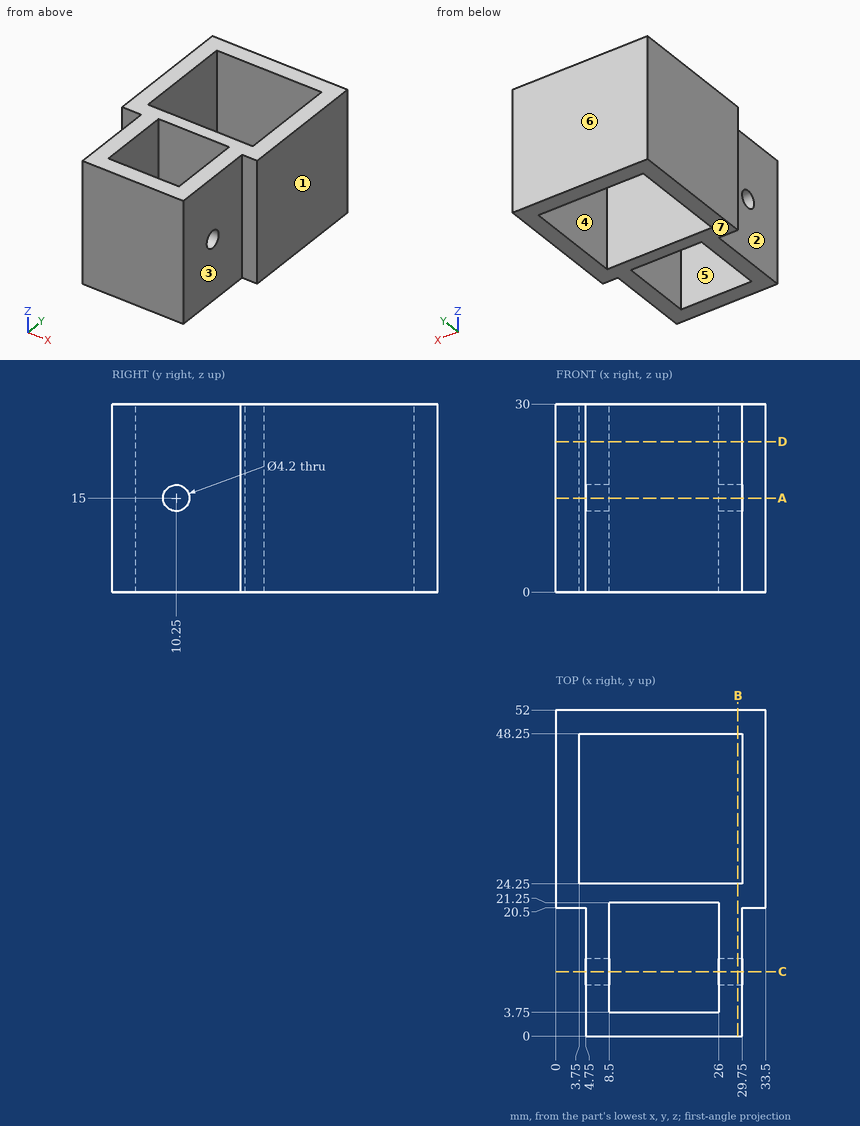
The figure shows three views and two pictorial views of one solid part (mm, origin at its lowest corner). Answer the questions. A direction names the side the tool comes from. Give positions to 0.01 mm unless a question says otherwise; leave off trailing zeros. Order: outer loops, then holes, each group sorted by start corner. A loop starts at its lowest first (then second) coordinate and runs counter-clockwise, first axis right, second up. Notation, with made-up numbers: M -6,-23 L 0,-23 A24 ccw 0,14 Z; hole C -38,5 d10. An arc over 180 degrees is marked long. Return JSON: item names as keys, results as strings.
1) Straight lines are drawn through the part: line 1 along Y through (x, z) = (10.5, 2.25); line 2 along X through (y, z) = (44.5, 27.5); line 3 along Z through (x, y) = (28.6, 10.25). For each, find the intervals that lie inside material, in ascending order. Write a range as [from, to].
Resolved:
{"line 1": "[0, 3.75], [21.25, 24.25], [48.25, 52]", "line 2": "[0, 3.75], [29.75, 33.5]", "line 3": "[0, 12.9], [17.1, 30]"}
2) Section D-D, the plane z = 24 is taken. Write down the section's boundary in (x, y), plus the area to 4 significant figures.
Resolved:
{"outline": "M 0,20.5 L 4.75,20.5 L 4.75,0 L 29.75,0 L 29.75,20.5 L 33.5,20.5 L 33.5,52 L 0,52 Z; hole M 3.75,24.25 L 29.75,24.25 L 29.75,48.25 L 3.75,48.25 Z; hole M 8.5,3.75 L 26,3.75 L 26,21.25 L 8.5,21.25 Z", "area": "637.5 mm^2"}
3) For a pull along Y with two mould halves and no side action, classify the marked faces 5, 6 and 7 as +Y half, -Y half, draft (parallel to the pull), parting line (faces both ways), or undercut.
Resolved:
{"face 5": "undercut", "face 6": "+Y half", "face 7": "draft"}
4) Section A-A, the plane z = 15 is taken. Write down the section's boundary in (x, y), plus the area to 3 significant figures.
Resolved:
{"outline": "M 0,20.5 L 4.75,20.5 L 4.75,12.35 L 8.5,12.35 L 8.5,21.25 L 26,21.25 L 26,12.35 L 29.75,12.35 L 29.75,20.5 L 33.5,20.5 L 33.5,52 L 0,52 Z; M 4.75,0 L 29.75,0 L 29.75,8.15 L 26,8.15 L 26,3.75 L 8.5,3.75 L 8.5,8.15 L 4.75,8.15 Z; hole M 3.75,24.25 L 29.75,24.25 L 29.75,48.25 L 3.75,48.25 Z", "area": "606 mm^2"}
5) A tool of negligible diameter and unlimited length cuts with its end or side. For the marked faces 1, 2, 3 and 4, from which of +Z, -Z, +X, -X, +Y, -Y can it reach the whole face along a straight path? Write none if from no direction.
Resolved:
{"face 1": "+Z, -Z, +X, +Y, -Y", "face 2": "+Z, -Z, -X, -Y", "face 3": "+Z, -Z, +X, -Y", "face 4": "+Z, -Z"}
6) Each of these flat-tipped pins is pushed along its axis until it touches: pin 1 (4 mm diameter, centred on y = 45, z = 13, fed in from -X); pin 2 (6.5 mm diameter, centred on y = 10.25, z = 15, fed in from +X); pin 3 (5 mm diameter, centred on y = 14.5, z = 13.5, fed in from -X); pin 4 (1.1 mm diameter, centred on x = 32, z = 12.5, fed in from -Y). Where does it stop, or does it pass through?
Resolved:
{"pin 1": "x = 0", "pin 2": "x = 29.75", "pin 3": "x = 4.75", "pin 4": "y = 20.5"}
7) Section B-B, the plane x = 29 is taken. Write down the section's boundary in (y, z), plus the area to 3 significant figures.
Resolved:
{"outline": "M 0,0 L 24.25,0 L 24.25,30 L 0,30 Z; M 48.25,0 L 52,0 L 52,30 L 48.25,30 Z; hole C 10.25,15 d4.2", "area": "826 mm^2"}
8) Section C-C, the plane y = 10.25 is taken. Write down the section's boundary in (x, z), plus the area to 4 significant figures.
Resolved:
{"outline": "M 4.75,0 L 8.5,0 L 8.5,12.9 L 4.75,12.9 Z; M 4.75,17.1 L 8.5,17.1 L 8.5,30 L 4.75,30 Z; M 26,0 L 29.75,0 L 29.75,12.9 L 26,12.9 Z; M 26,17.1 L 29.75,17.1 L 29.75,30 L 26,30 Z", "area": "193.5 mm^2"}
